```python
from build123d import *

# Parameters (mm, degrees)
SKETCH1_R           = 2.75
BOSS_EXTRUDE1_DEPTH = 2
FILLET1_R           = 1


with BuildPart() as part:
    # Sketch1 → Boss-Extrude1 (new body, symmetric)
    with BuildSketch(Plane.XY):
        Polygon((0, 0), (0, 59), (19, 59), (59, 19), (59, 0), align=None)
        with Locations((9.5, 9.5)):
            Circle(SKETCH1_R, mode=Mode.SUBTRACT)
        with Locations((29.5, 9.5)):
            Circle(SKETCH1_R, mode=Mode.SUBTRACT)
        with Locations((49.5, 9.5)):
            Circle(SKETCH1_R, mode=Mode.SUBTRACT)
        with Locations((9.5, 29.5)):
            Circle(SKETCH1_R, mode=Mode.SUBTRACT)
        with Locations((9.5, 49.5)):
            Circle(SKETCH1_R, mode=Mode.SUBTRACT)
    extrude(amount=BOSS_EXTRUDE1_DEPTH, both=True)

    # Fillet1
    fillet1_edges = [part.edges().sort_by_distance(p)[0] for p in [
        (39, 39, 2),
        (9.5, 59, 2),
        (0, 29.5, 2),
        (29.5, 0, 2),
        (59, 9.5, 2),
        (0, 0, 0),
        (0, 59, 0),
        (19, 59, 0),
        (59, 19, 0),
        (59, 0, 0),
    ]]
    fillet(fillet1_edges, radius=FILLET1_R)


solid = part.part
```
Read the model definition and answer for the solid it produces. Units are mm, in the model's axes. Give positions to 0.01 mm unless a question says otherwise; leave off trailing zeros. Order: outer loops, then holes, each group sorted by start corner. A loop starts at its lowest first (then second) coordinate and runs counter-clockwise, first axis right, second up.
(1) For a pull along Y with two mould halves and no side action, classify faces 1 (the flat face through (30, 0, 0)), 2 (the flat face through (23, 23, -2)), 3 (the cylindrical face through (9.142, 52.227, -0.028)) as released by +Y, released by -Y, zero draft, split by the parting line, or undercut.
(2) Straight lines are drawn through the part: L1, parallel to Y at x = 9.5, z = 0.9; L2, parallel to X at y = 10, z = 0.4; L3, parallel to Y at x = 49.5, z = 1.1. For each, find the intervals that lie inside material, in ascending order.
(3) Find section A-A (x = 9.5). Give the vertices of the cut face in (y, z), plus the area to 3 significant figures.
(4) Find section C-C (z = -0.65). Give the vertices of the cut face in (x, y).
(5) Given pin 1 (3.5 mm diameter, centred on x = 49.5, y = 9.5, fed in from -Z), flat-ended and moving along its own axis, determine where the tip first touches the part or whether it passes through.
Result sheet:
1. face 1: released by -Y
1. face 2: zero draft
1. face 3: undercut
2. L1: y = 0 to 6.75, 12.25 to 26.75, 32.25 to 46.75, 52.25 to 59
2. L2: x = 0 to 6.8, 12.2 to 26.8, 32.2 to 46.8, 52.2 to 59
2. L3: y = 0.01 to 6.75, 12.25 to 28.49
3. outline: (0, -2) - (6.75, -2) - (6.75, 2) - (1, 2) arc R1 ccw to (0, 1) - close; (12.25, -2) - (26.75, -2) - (26.75, 2) - (12.25, 2) - close; (32.25, -2) - (46.75, -2) - (46.75, 2) - (32.25, 2) - close; (52.25, -2) - (59, -2) - (59, 1) arc R1 ccw to (58, 2) - (52.25, 2) - close
3. area: 170 mm2
4. outline: (0, 1) arc R1 ccw to (1, 0) - (58, 0) arc R1 ccw to (59, 1) - (59, 18.59) arc R1 ccw to (58.71, 19.29) - (19.29, 58.71) arc R1 ccw to (18.59, 59) - (1, 59) arc R1 ccw to (0, 58) - close; hole circle Ø5.5 at (9.5, 9.5); hole circle Ø5.5 at (9.5, 29.5); hole circle Ø5.5 at (9.5, 49.5); hole circle Ø5.5 at (29.5, 9.5); hole circle Ø5.5 at (49.5, 9.5)
5. pin 1: passes through
